Can you work these out from the model? Positions are in its coordinate system, mm. Face numbers are marked on the shaded views. A direction names the side the tool comes from. Coordinates: 2 decimals unless noted, no trailing zeros. Order: outer loops, then holes, each group sorted by start corner. A loop starts at its lowest first (then second) coordinate and runs counter-clockwise, first axis right, second up. Notation, with made-up numbers: (74.25, 41.25) -> (93.25, 41.25) arc R18 cw to (93.25, 47.25) -> close; hole circle Ø5 at (-9.75, 81). An arc over 180 degrees is marked (long way). Answer as a JSON object with one key per item and string values. Group by question number.
(1) I want a section at A-A, the plane z = 2.5. List the corners of the cut face in (x, y) for me, plus the area to 3 significant figures.
(2) I need wall thicknesses on line 1 (Z direction, x = 0.5, y = 3.5); line 2 (X direction, y = 1.5, z = 1.5); line 3 (Y direction, x = -2.75, z = 3). Which ranges of each line are inside material? Lowest first, please.
(3) If we mould it in two halves opening along Y, with no side actions, what happens to the marked faces 5, 6 and 7? For each: pulls with the +Y half, pulls with the -Y half, needs draft (parallel to the pull), parting line crosses it, or undercut.
(4) For pin 1 (3.5 mm diameter, centred on y = -3.5, z = 1.5, fed in from +X); pin 2 (3.5 mm diameter, centred on x = 3, z = 2.5, fed in from -Y); pin 3 (3.5 mm diameter, centred on y = 2.5, z = 1, fed in from +X), each with a flat end and sliding along its axis, tell me the tip position at first contact or that it passes through.
(5) I want a section at D-D, the plane z = 5.75. List the corners of the cut face in (x, y) for me.
(6) Which directions (+Z, -Z, +X, -X, +Y, -Y) give clear straight access to the entire face, cutting with the end or side of a thin tool? Please do the marked faces 1, 2, 3 and 4.
(7) I want a section at B-B, the plane x = 0. List the corners of the cut face in (y, z) for me.
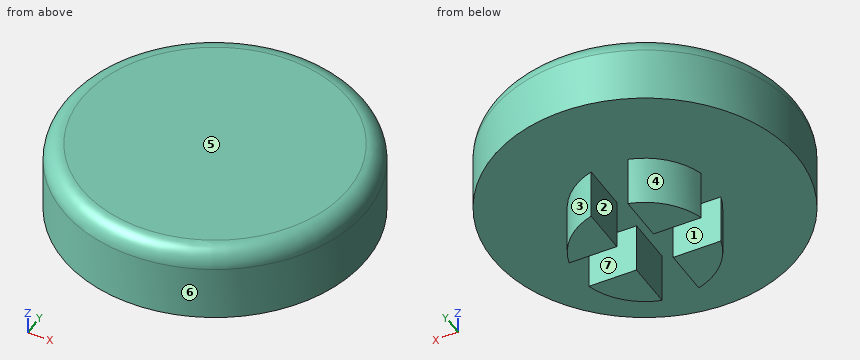
from build123d import *

# Parameters (mm, degrees)
F0_R     = 4.75
F1_DEPTH = 3.5
F2_R     = 10.5
F2_R_2   = 4.75
F3_DEPTH = 5.08
F4_R     = 1.27
F6_DEPTH = 25.4


with BuildPart() as f1:
    # F0 (on Top) → F1 (new body)
    with BuildSketch(Plane.XY):
        Circle(F0_R)
    extrude(amount=F1_DEPTH)

    # F2 (on face) → F3 (join)
    with BuildSketch(Plane.XY.offset(3.5)):
        Circle(F2_R)
        Circle(F2_R_2, mode=Mode.SUBTRACT)
        Circle(F2_R_2)
    extrude(amount=F3_DEPTH)

    # F4
    f4_edges = [f1.edges().sort_by_distance(p)[0] for p in [
        (-10.5, 0, 8.58),
    ]]
    fillet(f4_edges, radius=F4_R)

    # F5 (on face) → F6 (cut)
    with BuildSketch(Plane(origin=(0, 0, 3.5), x_dir=(1, 0, 0), z_dir=(0, 0, -1))):
        Polygon((1.27, 1.27), (1.27, 0), (1.27, -1.27), (10.422912261, -1.27), (10.422912261, 1.27), align=None)
        Polygon((1.27, -1.27), (1.27, 0), (1.27, 1.27), (0, 1.27), (-1.27, 1.27), (-1.27, 0), (-1.27, -1.27), (0, -1.27), align=None)
        Polygon((1.27, -10.422912261), (1.27, -1.27), (0, -1.27), (-1.27, -1.27), (-1.27, -10.422912261), align=None)
        Polygon((0, 1.27), (1.27, 1.27), (1.27, 10.422912261), (-1.27, 10.422912261), (-1.27, 1.27), align=None)
        Polygon((-10.422912261, -1.27), (-1.27, -1.27), (-1.27, 0), (-1.27, 1.27), (-10.422912261, 1.27), align=None)
    extrude(amount=F6_DEPTH, mode=Mode.SUBTRACT)


solid = f1.part
Computed values:
{
 "1": {"outline": "(-4.58, -1.27) arc R4.75 ccw to (-1.27, -4.58) -> (-1.27, -1.27) -> close; (-4.58, 1.27) -> (-1.27, 1.27) -> (-1.27, 4.58) arc R4.75 ccw to start; (1.27, -4.58) arc R4.75 ccw to (4.58, -1.27) -> (1.27, -1.27) -> close; (1.27, 1.27) -> (4.58, 1.27) arc R4.75 ccw to (1.27, 4.58) -> close", "area": "29.7 mm2"},
 "2": {"line 1": "z = 3.5 to 8.58", "line 2": "x = -4.51 to -1.27, 1.27 to 4.51", "line 3": "y = -3.87 to -1.27, 1.27 to 3.87"},
 "3": {"face 5": "needs draft", "face 6": "parting line crosses it", "face 7": "undercut"},
 "4": {"pin 1": "stops at x = 4.42", "pin 2": "stops at y = -10.38", "pin 3": "stops at x = 4.58"},
 "5": {"outline": "circle Ø21 at (0, 0)"},
 "6": {"face 1": "-Z, +X, -X", "face 2": "-Z, +Y, -Y", "face 3": "-Z, +X, +Y", "face 4": "-Z, -X, +Y"},
 "7": {"outline": "(-10.5, 3.5) -> (10.5, 3.5) -> (10.5, 7.31) arc R1.27 ccw to (9.23, 8.58) -> (-9.23, 8.58) arc R1.27 ccw to (-10.5, 7.31) -> close"}
}
